Verification items for this drawing (mm, ordinates from the low corner). A direction names the side the tool comes from. Coordinates: 2 decimals unless noted, no trailing zeros. Order: outer loops, then holes, each group sorted by start corner. A loop starts at its lowest first (then second) coordinate and runs counter-clockwise, first axis right, second up. Notation, with made-up numbers: M 22.5,-6 L 55.5,-6 A5 cw 55.5,3 Z; hole C 27,15.25 d10. An arc over 180 degrees is marked long. Write item = value, one per line.
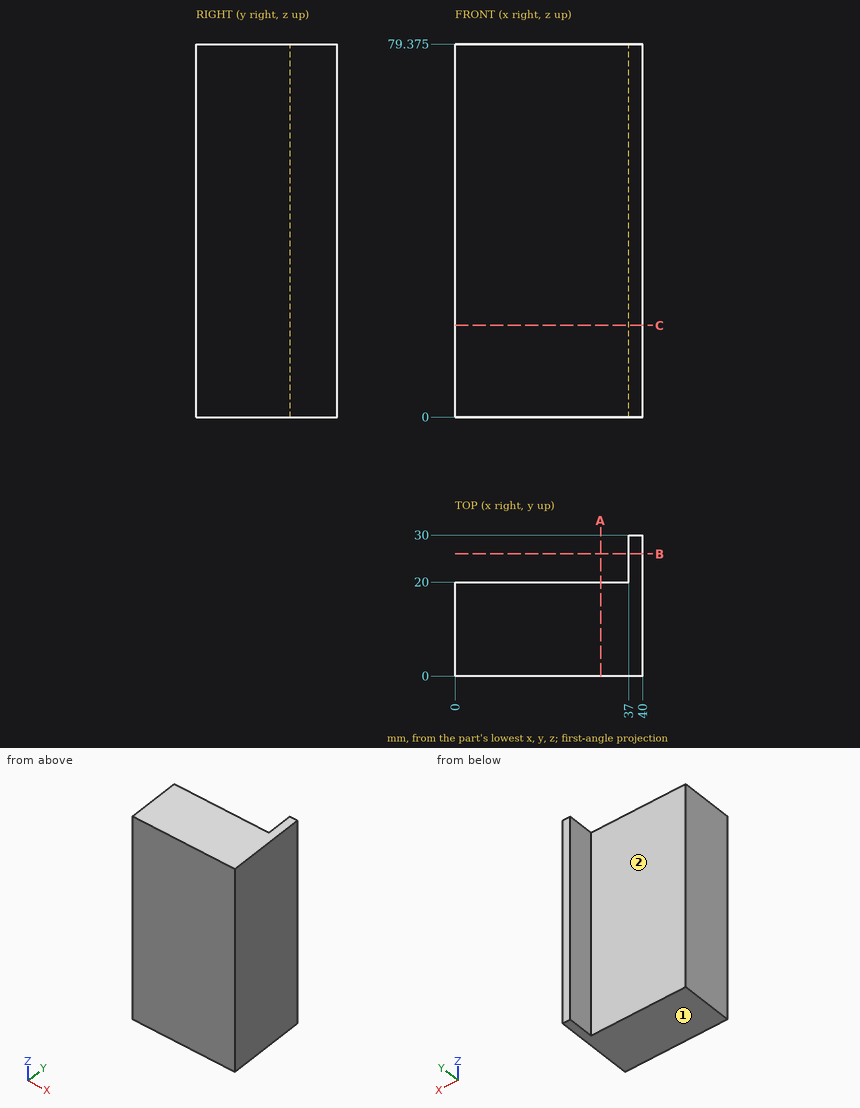
Item 1: Sectioned sample at C-C, the plane z = 19.5. Enter the section's corners in (x, y), then the cut area to 3 significant figures.
Report:
outline = M 0,0 L 40,0 L 40,30 L 37,30 L 37,20 L 0,20 Z
area = 830 mm^2
Item 2: Gauge pin test, flat ends, axial feed: pin 1 (5 mm diameter, centred on y = 25.5, z = 44, fed in from -X); pin 2 (12 mm diameter, centred on x = 17.5, z = 63.5, fed in from +Y). Record the tip position at first contact, or that the pin passes through.
Report:
pin_1 = 37
pin_2 = 20
Item 3: Sectioned sample at B-B, the plane y = 26. Enter the section's corners in (x, z) (3 decimals), then the cut area to 3 significant figures.
Report:
outline = M 37,0 L 40,0 L 40,79.375 L 37,79.375 Z
area = 238 mm^2
Item 4: Tool access check on the marked faces 1 and 2. Record the directions out of +Z, -Z, +X, -X, +Y, -Y that give a thin tool (end or side, any length) a straight path to the whole face; none if there is none.
Report:
face_1 = -Z, +X, -X, +Y, -Y
face_2 = +Z, -Z, -X, +Y
Item 5: Scan lines: L1, parallel to X at y = 21.25, z = 54; L2, parallel to Y at x = 26.5, z = 51. Record each from-to range of solid material in increasing order. Write a range as from..to.
Report:
L1 = 37..40
L2 = 0..20
Item 6: Sectioned sample at A-A, the plane x = 31. Enter the section's corners in (y, z) (3 decimals).
Report:
outline = M 0,0 L 20,0 L 20,79.375 L 0,79.375 Z
